from build123d import *

# Parameters (mm, degrees)
F0_R           = 17.35
F0_R_2         = 16.35
F1_DEPTH       = 17.5
F2_W           = 4
F2_H           = 5
F5_D           = 12
F5_DEPTH       = 30
F5_CSINK_D     = 32
F5_CSINK_ANGLE = 82
F5_TIP         = 3.6051637142
F6_DEPTH       = 18
F7_R           = 4
F8_DEPTH       = 17.5
F10_R          = 4
F11_DEPTH      = 17.5
F13_DEPTH      = 4


with BuildPart() as f1:
    # F0 (on Front) → F1 (new body, symmetric)
    with BuildSketch(Plane.XZ):
        Circle(F0_R)
        Circle(F0_R_2, mode=Mode.SUBTRACT)
        Circle(F0_R_2)
    extrude(amount=F1_DEPTH, both=True)

    # F2 (on Right) → F3 (revolve, cut)
    with BuildSketch(Plane.YZ):
        with Locations((-11.5, 17.9)):
            Rectangle(F2_W, F2_H)
        with Locations((11.5, 17.9)):
            Rectangle(F2_W, F2_H)
    revolve(axis=Axis((0, 0, 0), (0, -1, 0)), mode=Mode.SUBTRACT)

    # F5
    with Locations(Plane.XZ.offset(17.5)):
        with Locations((0, 0)):
            CounterSinkHole(F5_D / 2, F5_CSINK_D / 2, depth=F5_DEPTH, counter_sink_angle=F5_CSINK_ANGLE)
            with Locations((0, 0, -(F5_DEPTH + F5_TIP / 2))):  # 118° drill point
                Cone(0, F5_D / 2, F5_TIP, mode=Mode.SUBTRACT)

    # F4 (on face) → F6 (cut)
    with BuildSketch(Plane.XZ.offset(17.5)):
        with BuildLine():
            ThreePointArc((-4.472135955, -4), (-6, 0), (-4.472135955, 4))
            Line((-4.472135955, 4), (-10, 4))
            Line((-10, 4), (-10, -4))
            Line((-10, -4), (-4.472135955, -4))
        make_face()
        with BuildLine():
            ThreePointArc((4.472135955, 4), (5.6050341538, 2.1409325386), (6, 0))
            ThreePointArc((6, 0), (5.6050341538, -2.1409325386), (4.472135955, -4))
            Line((4.472135955, -4), (10, -4))
            Line((10, -4), (10, 4))
            Line((10, 4), (4.472135955, 4))
        make_face()
    extrude(amount=-F6_DEPTH, mode=Mode.SUBTRACT)

    # F7 (on Right) → F8 (cut, symmetric)
    with BuildSketch(Plane.YZ):
        Circle(F7_R)
    extrude(amount=F8_DEPTH, both=True, mode=Mode.SUBTRACT)

    # F10 (on face) → F11 (cut, symmetric)
    with BuildSketch(Plane(origin=(0, 0, 0), x_dir=(0, 1, 0), z_dir=(0.7071067812, 0, -0.7071067812))):
        Circle(F10_R)
    extrude(amount=F11_DEPTH, both=True, mode=Mode.SUBTRACT)

    # F12 (on Front) → F13 (cut, symmetric)
    with BuildSketch(Plane.XZ):
        with BuildLine():
            Line((-17.35, 0), (0, 0))
            Line((0, 0), (-12.2683026536, 12.2683026536))
            ThreePointArc((-12.2683026536, 12.2683026536), (-13.6092339975, 10.7615635481), (-14.7662347124, 9.1093804629))
            ThreePointArc((-14.7662347124, 9.1093804629), (-16.6915648197, 4.7343599219), (-17.35, 0))
        make_face()
        with BuildLine():
            ThreePointArc((14.7662347124, -9.1093804629), (16.6915648197, -4.7343599219), (17.35, 0))
            Line((17.35, 0), (0, 0))
            Line((0, 0), (12.2683026536, -12.2683026536))
            ThreePointArc((12.2683026536, -12.2683026536), (13.6092339975, -10.7615635481), (14.7662347124, -9.1093804629))
        make_face()
    extrude(amount=F13_DEPTH, both=True, mode=Mode.SUBTRACT)


solid = f1.part
Check sheet for the modelled part. Datum: model origin and axes. Units: mm. A direction names the side the tool comes from. Coordinates: 2 decimals unless noted, no trailing zeros. Loops run counter-clockwise (first coordinate to the right, second up) from the corner with the lowest first, then second, coordinate; pieces in that order, holes last. Notation, with made-up numbers: (60.5, 31) -> (68.5, 31) arc R23 cw to (68.5, 46) -> close; hole circle Ø4 at (63, -13). An arc over 180 degrees is marked (long way). Answer in a Markdown table with one row per item.
1. Sectioned sample at C-C, the plane y = 15. Record the boundary of the cut face in (x, z), then the cut area to 3 significant figures.
Check values:
| item | result |
|---|---|
| outline | circle Ø34.7 at (0, 0); hole circle Ø3.68 at (0, 0) |
| area | 935 mm2 |
2. Go/stop test with flat-tipped pins: pin 1 (1.5 mm diameter, centred on x = -7.5, y = 12, fed in from +Z); pin 2 (3.5 mm diameter, centred on x = -12, z = 3, fed in from -Y); pin 3 (8 mm diameter, centred on y = -8, z = 13, fed in from -X). Record where each tip stops, or that it passes through.
Check values:
| item | result |
|---|---|
| pin 1 | stops at z = 13.84 |
| pin 2 | stops at y = -15.34 |
| pin 3 | stops at x = -14.83 |
3. Release check for a two-part mould opening along Z. For faces 4 (the face through (-2.259, 15.472, 17.202)), 5 (the face through (14, -13.5, 7)), 6 (the face through (11, 4, -5)) record: released by +Z, released by -Z, zero draft, split by the parting line, or undercut.
Check values:
| item | result |
|---|---|
| face 4 | split by the parting line |
| face 5 | zero draft |
| face 6 | undercut |
4. Sectioned sample at A-A, the plane y = -8. Record the boundary of the cut face in (x, z), then the cut area to 3 significant figures.
Check values:
| item | result |
|---|---|
| outline | circle Ø34.7 at (0, 0); hole (-10, -4) -> (-6.63, -4) arc R7.74 ccw to (6.63, -4) -> (10, -4) -> (10, 4) -> (6.63, 4) arc R7.74 ccw to (-6.63, 4) -> (-10, 4) -> close |
| area | 716 mm2 |
5. Material ranges on line 1 along Z through (x, y) = (0, 4.5); line 2 along Y through (x, z) = (-15, -5.5); line 3 along Y through (x, z) = (-10, -12), recorded low to high. Write a range as [from, to].
Check values:
| item | result |
|---|---|
| line 1 | z = [-17.35, -6], [6, 17.35] |
| line 2 | y = [-17.47, -13.5], [-9.5, 9.5], [13.5, 17.5] |
| line 3 | y = [-17.06, -13.5], [-9.5, 9.5], [13.5, 17.5] |
6. Sectioned sample at B-B, the plane y = 3. Record the boundary of the cut face in (x, z), then the cut area to 3 significant figures.
Check values:
| item | result |
|---|---|
| outline | (-17.15, -2.65) arc R17.35 ccw to (10.25, -14) -> (1.94, -5.68) arc R6 cw to (-5.39, -2.65) -> close; (-10.25, 14) -> (-1.94, 5.68) arc R6 cw to (5.39, 2.65) -> (17.15, 2.65) arc R17.35 ccw to start |
| area | 503 mm2 |
7. Access from +Z, -Z, +X, -X, +Y, -Y to the whole of each face (thin tool, end or side, straight path). Record for faces 1 (the face through (4.951, -0.088, -10.607)), 2 (the face through (-8, -7, 4)), 3 (the face through (-12.263, 1.285, -3.788)).
Check values:
| item | result |
|---|---|
| face 1 | +X |
| face 2 | -Y |
| face 3 | +X, -X |
